from build123d import *

# Parameters (mm, degrees)
BOSS_EXTRUDE1_DEPTH = 16.2
SKETCH2_R           = 7.5
BOSS_EXTRUDE2_DEPTH = 7
SKETCH3_R           = 4
BOSS_EXTRUDE3_DEPTH = 4
CHAMFER1_SIZE       = 0.6
SKETCH4_R           = 2.5
CUT_EXTRUDE1_DEPTH  = 20


with BuildPart() as part:
    # Sketch1 → Boss-Extrude1 (new body)
    with BuildSketch(Plane.XY):
        Polygon((2.857883832, -4.95), (5.715767665, 0), (2.857883832, 4.95), (-2.857883832, 4.95), (-5.715767665, 0), (-2.857883832, -4.95), align=None)
    extrude(amount=BOSS_EXTRUDE1_DEPTH)

    # Sketch2 → Boss-Extrude2 (add)
    with BuildSketch(Plane.XY):
        Circle(SKETCH2_R)
    extrude(amount=-BOSS_EXTRUDE2_DEPTH)

    # Sketch3 → Boss-Extrude3 (add)
    with BuildSketch(Plane(origin=(0, 0, -7), x_dir=(-1, 0, 0), z_dir=(0, 0, -1))):
        with BuildLine():
            Line((-18, 9), (18, 9))
            ThreePointArc((18, 9), (27, 0), (18, -9))
            Line((18, -9), (-18, -9))
            ThreePointArc((-18, -9), (-27, 0), (-18, 9))
        make_face()
        with Locations((-18, 0)):
            Circle(SKETCH3_R, mode=Mode.SUBTRACT)
        with Locations((18, 0)):
            Circle(SKETCH3_R, mode=Mode.SUBTRACT)
    extrude(amount=BOSS_EXTRUDE3_DEPTH)

    # Chamfer1
    chamfer1_edges = [part.edges().sort_by_distance(p)[0] for p in [
        (4.286825749, 2.475, 16.2),
        (0, 4.95, 16.2),
        (-7.5, 0, 0),
        (-4.286825749, 2.475, 16.2),
        (-4.286825749, -2.475, 16.2),
        (27, 0, -11),
        (0, -9, -11),
        (-27, 0, -11),
        (0, 9, -11),
        (22, 0, -7),
        (-14, 0, -7),
        (27, 0, -7),
        (0, -9, -7),
        (-27, 0, -7),
        (0, 9, -7),
        (22, 0, -11),
        (-14, 0, -11),
        (0, -4.95, 16.2),
        (4.286825749, -2.475, 16.2),
    ]]
    chamfer(chamfer1_edges, length=CHAMFER1_SIZE)

    # Sketch4 → Cut-Extrude1 (cut)
    with BuildSketch(Plane.XY.offset(16.2)):
        Circle(SKETCH4_R)
    extrude(amount=-CUT_EXTRUDE1_DEPTH, mode=Mode.SUBTRACT)


solid = part.part
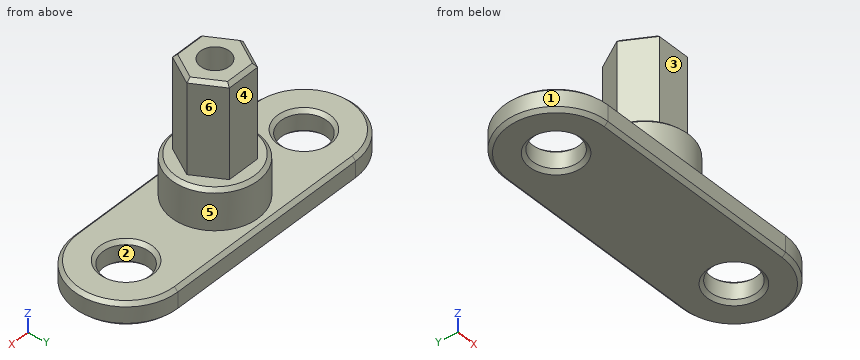
The model under review builds one solid part; all positions refer to its coordinate system, in mm. Face numbers are marked on the shaded views. A direction names the side the tool comes from. Give positions to 0.01 mm unless a question says otherwise; leave off trailing zeros. Write each loop counter-clockwise with the first axis right and the second up, starting at its lowest first coordinate (ties: lowest second). Pieces come first, ordered by that corner, then holes.
1. Add section C-C, the plane y = 1.5. Count the separate pieces of the cut face and the enclosed holes in it, plus the area to 3 significant figures.
2. For P1, Ø8, axis at y = 1.5, z = -1.5, coming from the -X side; P2, Ø3, axis at x = 0, z = 9, coming from the -Y side; P3, Ø5, axis at y = 4, z = -3, coming from the -X side, all flat-tipped, find the tip position at first contact; note any pin that passes through.
3. Add section B-B, the plane x = 0. Write out the cut boundary in (y, z), plus the area to 3 significant figures.
4. Tool access review of the marked faces 4, 5 and 6: name each direction out of +Z, -Z, +X, -X, +Y, -Y from which nothing blocks a thin tool from reaching the whole face with its end or side.
5. Draft analysis for pull direction X (two halves, no side actions). For the marked faces 1, 2 and 3, state which applies: +X half, -X half, draft (parallel to the pull), parting line (faces both ways), or undercut.
6. Add section A-A, the plane z = 8.5. Write out the cut boundary in (x, y), plus the area to 3 significant figures.
7. Wall thickness on L1, parallel to Y at x = 0, z = 11.25; L2, parallel to Y at x = -18, z = -8.4; L3, parallel to Z at x = 20.5, y = -6: over which ranges is each line inside the solid? List them lowest first.
Worked answers:
1. separate pieces: 3
1. enclosed holes: 0
1. area: 333 mm2
2. P1: stops at x = -7.5
2. P2: stops at y = -4.95
2. P3: stops at x = -7.35
3. outline: (-9, -10.4) - (-8.4, -11) - (8.4, -11) - (9, -10.4) - (9, -7.6) - (8.4, -7) - (7.5, -7) - (7.5, -0.6) - (6.9, 0) - (4.95, 0) - (4.95, 15.6) - (4.35, 16.2) - (2.5, 16.2) - (2.5, -3.8) - (-2.5, -3.8) - (-2.5, 16.2) - (-4.35, 16.2) - (-4.95, 15.6) - (-4.95, 0) - (-6.9, 0) - (-7.5, -0.6) - (-7.5, -7) - (-8.4, -7) - (-9, -7.6) - close
3. area: 236 mm2
4. face 4: +Z, +X, -X, +Y
4. face 5: +Z
4. face 6: +Z, +X, +Y
5. face 1: -X half
5. face 2: undercut
5. face 3: draft
6. outline: (-5.72, 0) - (-2.86, -4.95) - (2.86, -4.95) - (5.72, 0) - (2.86, 4.95) - (-2.86, 4.95) - close; hole circle Ø5 at (0, 0)
6. area: 65.2 mm2
7. L1: y = -4.95 to -2.5, 2.5 to 4.95
7. L2: y = -9 to -4, 4 to 9
7. L3: z = -11 to -7
